Autodesk Fusion 360 part; units mm, degrees
sketch "Sketch1" plane through (0, 0, 0) normal (0, 0, 1) x (1, 0, 0)
  line L0 (-24, -23) -> (24, -23)
  line L1 (24, -23) -> (24, 23)
  line L2 (24, 23) -> (-24, 23)
  line L3 (-24, 23) -> (-24, -23)
  dimension "d1" = 48
  dimension "d2" = 46
  dimension "d3" = 24
  dimension "d4" = 23
extrude "Extrude1" add sketch "Sketch1" along normal blind 55
sketch "Sketch2" plane through (0, -23, 0) normal (0, -1, 0) x (1, 0, 0)
  line L0 (-24, 0) -> (24, 0)
  line L1 (24, 0) -> (24, 55)
  line L2 (24, 55) -> (-24, 55)
  line L3 (-24, 55) -> (-24, 0)
  line L4 (-20, 51) -> (20, 51)
  line L5 (20, 51) -> (20, 4)
  line L6 (20, 4) -> (-20, 4)
  line L7 (-20, 4) -> (-20, 51)
  dimension "d7" = 40
  dimension "d8" = 20
  dimension "d10" = 4
  dimension "d58" = 4
extrude "Extrude2" cut sketch "Sketch2" against normal blind 42 contours L4 L5 L6 L7
sketch "Sketch4" plane through (0, 0, 55) normal (0, 0, 1) x (-1, 0, 0)
  line L0 (24, -23) -> (24, 23)
  line L1 (24, 23) -> (-24, 23)
  line L2 (-24, 23) -> (-24, -23)
  line L3 (-24, -23) -> (24, -23)
  circle A0 centre (0, 0) radius 6
  dimension "d23" = 12
hole "Hole1" at (0, 0, 55) direction (0, 0, -1) diameter 12 depth 4 tip angle 118
sketch "Sketch5" plane through (0, 0, 55) normal (0, 0, 1) x (-1, 0, 0)
  circle A0 centre (0, 0) radius 6
  line L0 (24, -23) -> (24, 23)
  line L1 (24, 23) -> (-24, 23)
  line L2 (-24, 23) -> (-24, -23)
  line L3 (-24, -23) -> (24, -23)
  circle A1 centre (-8.8388, -8.8388) radius 1.5
  point P0 (8.8388, -8.8388)
  point P1 (8.8388, 8.8388)
  point P2 (-8.8388, 8.8388)
  dimension "d27" = 12.5
  dimension "d28" = 3
  dimension "d30" = 360
hole "Hole2" at (8.8388, 8.8388, 55) at (-8.8388, 8.8388, 55) at (-8.8388, -8.8388, 55) at (8.8388, -8.8388, 55) direction (0, 0, -1) diameter 4 depth 4 tip angle 118 countersink diameter 6 countersink angle 90
sketch "Sketch7" plane through (0, 0, 0) normal (0, 0, -1) x (1, 0, 0)
  line L0 (-24, 23) -> (-24, -23)
  line L1 (-24, -23) -> (24, -23)
  line L2 (24, -23) -> (24, 23)
  line L3 (24, 23) -> (-24, 23)
  circle A0 centre (0, 0) radius 5
  circle A1 centre (5.6569, -5.6569) radius 2
  circle A2 centre (6.7175, 6.7175) radius 2
  circle A3 centre (-6.7175, -6.7175) radius 2
  circle A4 centre (-5.6569, 5.6569) radius 2
  dimension "d45" = 10
  dimension "d67" = 4
  dimension "d68" = 4
  dimension "d69" = 9.5
  dimension "d70" = 8
  dimension "d71" = 17.3431
  dimension "d72" = 16.2825
  dimension "d74" = 360
extrude "Extrude4" cut sketch "Sketch7" against normal blind 4 contours A0 | A1 | A2 | A3 | A4
sketch "Sketch8" plane through (0, 0, 55) normal (0, 0, 1) x (-1, 0, 0)
  circle A0 centre (0, 0) radius 6
  line L0 (24, -23) -> (24, 23)
  line L1 (24, 23) -> (-24, 23)
  line L2 (-24, 23) -> (-24, -23)
  line L3 (-24, -23) -> (24, -23)
  ellipse E0 centre (0, 0) end of major axis (0, 8.5421) minor radius 3.3168
  line L4 (0, -8.5421) -> (0, 8.5421)
  line L5 (3.3168, 0) -> (-3.3168, 0)
  circle A1 centre (8.8388, 8.8388) radius 3
  circle A2 centre (-8.8388, -8.8388) radius 3
  circle A3 centre (8.8388, -8.8388) radius 3
  circle A4 centre (-8.8388, 8.8388) radius 3
extrude "Extrude5" cut sketch "Sketch8" against normal blind 4 contours A0 E0 | A0 E0
sketch "Sketch3" plane through (24, 0, 0) normal (1, 0, 0) x (0, 1, 0)
  line L0 (-21, 0) -> (23, 0)
  line L1 (23, 0) -> (23, 50)
  line L2 (23, 50) -> (-21, 50)
  line L3 (-11, 47) -> (-6, 47)
  line L4 (-6, 47) -> (-6, 8)
  line L5 (-6, 8) -> (-11, 8)
  line L6 (-11, 8) -> (-11, 47)
  line L7 (6, 47) -> (11, 47)
  line L8 (11, 47) -> (11, 8)
  line L9 (11, 8) -> (6, 8)
  line L10 (6, 8) -> (6, 47)
  line L11 (-23, 0) -> (23, 0)
  line L12 (23, 0) -> (23, 55)
  line L13 (23, 55) -> (-23, 55)
  line L14 (-23, 55) -> (-23, 0)
  line L15 (-23, 51) -> (-23, 4)
  point P0 (-23, 55)
  point P1 (23, 55)
  dimension "d16" = 8
  dimension "d20" = 12
  dimension "d60" = 8
  dimension "d75" = 5
  dimension "d76" = 5
  dimension "d97" = 12
  dimension "d100" = 8
  dimension "d101" = 8
extrude "Extrude6" cut sketch "Sketch3" against normal blind 48 contours L3 L4 L5 L6 | L7 L8 L9 L10
sketch "Sketch9" plane through (0, 23, 0) normal (0, 1, 0) x (-1, 0, 0)
  line L0 (-24, 0) -> (24, 0)
  line L1 (24, 0) -> (24, 55)
  line L2 (24, 55) -> (-24, 55)
  line L3 (-24, 55) -> (-24, 0)
  line L4 (-12, 47) -> (-7, 47)
  line L5 (-7, 47) -> (-7, 8)
  line L6 (-7, 8) -> (-12, 8)
  line L7 (-12, 8) -> (-12, 47)
  line L8 (7, 47) -> (12, 47)
  line L9 (12, 47) -> (12, 8)
  line L10 (12, 8) -> (7, 8)
  line L11 (7, 8) -> (7, 47)
  line L12 (-24, 0) -> (24, 0)
  dimension "d79" = 8
  dimension "d80" = 8
  dimension "d81" = 8
  dimension "d82" = 8
  dimension "d83" = 12
  dimension "d84" = 12
  dimension "d85" = 5
  dimension "d86" = 5
extrude "Extrude7" cut sketch "Sketch9" against normal blind 44 contours L4 L5 L6 L7 | L8 L9 L10 L11
fillet "Fillet2" radius 3.5 3 edges at (0, 19, 4) (-20, -2, 4) (20, -2, 4)
fillet "Fillet3" radius 2 24 edges at (22, 11, 8) (22, -6, 8) (-22, 11, 8) (-22, -6, 8) (22, 6, 8) (22, -11, 8) (22, -11, 47) (22, 6, 47) (22, 11, 47) (22, -6, 47) (-22, -6, 47) (-22, -11, 47) (-22, 6, 47) (-22, 11, 47) (-22, -11, 8) (-22, 6, 8) (-7, 21, 8) (12, 21, 8) (7, 21, 8) (-12, 21, 8) (12, 21, 47) (-7, 21, 47) (7, 21, 47) (-12, 21, 47)
fillet "Fillet4" radius 2 3 edges at (-20, -2, 51) (0, 19, 51) (20, -2, 51)
Source: CAD feature listing. Evaluate the final solid. Frame: model axes, mm. A direction names the side the tool comes from. Round coordinates to 2 decimals unless told otherwise and drop trailing zeros. Loops run counter-clockwise (first coordinate to the right, second up) from the corner with the lowest first, then second, coordinate; pieces in that order, holes last. Notation, with made-up numbers: M 73.25,61.5 L 95.25,61.5 A21 cw 95.25,71.5 Z; hole C -36.75,21.25 d1. An arc over 180 degrees is marked long. Return JSON: item names as keys, results as strings. Group by question number.
1. Section query C-C on x = 0. Output: boundary loops of the cut face in (y, z), and give its area (3 significant figures).
2. Pin query (flat end, axial travel): pin 1 (1.5 mm diameter, centred on x = -3, z = 21, fed in from -Y); pin 2 (8 mm diameter, centred on x = 0, y = 0, fed in from +Z); pin 3 (5 mm diameter, centred on x = -8.84, y = -8.84, fed in from +Z). Return the tip coordinate at first contact, or that it passes through.
3. Material intervals for line 1 along X through (y, z) = (-11.5, 47); line 2 along Y through (x, z) = (0, 1.95); line 3 along Z through (x, y) = (-10, -12), sorted ascending. Write a range as from..to.
4. Mould query, pull axis Y, two halves, no side actions, for faces 6 (the face through (21.97, 10.43, 8.6)), 7 (the face through (0, 23, 27)), 8 (the face through (0, -8, 51)). Classes: released by +Y, released by -Y, zero draft, split by the parting line, or undercut.
5. Reachability of faces 1 (the face through (-5.642, 5.031, 1.972)), 2 (the face through (22, 11, 28)), 3 (the face through (-24, 0, 27)), 4 (the face through (-12, 21, 28)), 5 (the face through (-3.4, -4, 4)) from +Z, -Z, +X, -X, +Y, -Y: full face, straight path, thin tool, end or side. Return the list, or none.
6. Section query A-A on z = 17. State how many separate pieces and enclosed holes the cut face has, and give its area (3 significant figures).
7. Section query B-B on y = 0. Output: boundary loops of the cut face in (x, z).
Checks:
{
 "1": {"outline": "M -23,0 L -5,0 L -5,4 L -23,4 Z; M -23,51 L -6,51 L -6,55 L -23,55 Z; M 5,0 L 23,0 L 23,55 L 6,55 L 6,51 L 17,51 A2 cw 19,49 L 19,7.5 A3.5 cw 15.5,4 L 5,4 Z", "area": "471 mm²"},
 "2": {"pin 1": "stops at y = 19", "pin 2": "passes through", "pin 3": "stops at z = 54.5"},
 "3": {"line 1": "x = -24..-20, 20..24", "line 2": "y = -23..-5, 5..23", "line 3": "z = 0..4, 51..55"},
 "4": {"face 6": "undercut", "face 7": "released by +Y", "face 8": "zero draft"},
 "5": {"face 1": "-Z", "face 2": "+X, -X", "face 3": "+Z, -Z, -X, +Y, -Y", "face 4": "+Y, -Y", "face 5": "-Y"},
 "6": {"separate pieces": "7", "enclosed holes": "0", "area": "408 mm²"},
 "7": {"outline": "M -24,0 L -5,0 L -5,4 L -16.5,4 A3.5 cw -20,7.5 L -20,49 A2 cw -18,51 L -6,51 L -6,55 L -24,55 Z; M 5,0 L 24,0 L 24,55 L 6,55 L 6,51 L 18,51 A2 cw 20,49 L 20,7.5 A3.5 cw 16.5,4 L 5,4 Z"}
}
